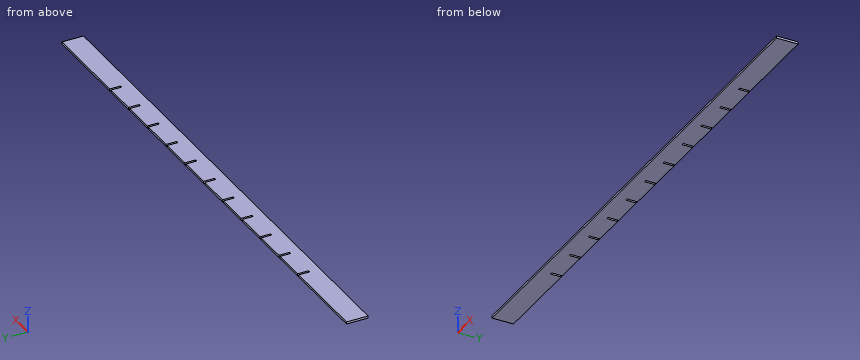
from build123d import *

# Parameters (mm, degrees)
ESQUISSE1_W                = 500
ESQUISSE1_H                = 20
BOSS_EXTRU_1_DEPTH         = 1
ESQUISSE2_W                = 2
ESQUISSE2_H                = 10
ENL_V_MAT_EXTRU_1_DEPTH    = 3
R_P_TITION_LIN_AIRE3_COUNT = 6
R_P_TITION_LIN_AIRE3_PITCH = 33
SYM_TRIE1_COPY_1_SKETCH_W  = 2
SYM_TRIE1_COPY_1_SKETCH_H  = 10
SYM_TRIE1_COPY_1_DEPTH     = 3
SYM_TRIE1_COPY_2_SKETCH_W  = 2
SYM_TRIE1_COPY_2_SKETCH_H  = 10
SYM_TRIE1_COPY_2_DEPTH     = 3
SYM_TRIE1_COPY_3_SKETCH_W  = 2
SYM_TRIE1_COPY_3_SKETCH_H  = 10
SYM_TRIE1_COPY_3_DEPTH     = 3
SYM_TRIE1_COPY_4_SKETCH_W  = 2
SYM_TRIE1_COPY_4_SKETCH_H  = 10
SYM_TRIE1_COPY_4_DEPTH     = 3
SYM_TRIE1_COPY_5_SKETCH_W  = 2
SYM_TRIE1_COPY_5_SKETCH_H  = 10
SYM_TRIE1_COPY_5_DEPTH     = 3
SYM_TRIE1_COPY_6_SKETCH_W  = 2
SYM_TRIE1_COPY_6_SKETCH_H  = 10
SYM_TRIE1_COPY_6_DEPTH     = 3


with BuildPart() as part:
    # Esquisse1 → Boss.-Extru.1 (new body, symmetric)
    with BuildSketch(Plane.XY):
        Rectangle(ESQUISSE1_W, ESQUISSE1_H)
    extrude(amount=BOSS_EXTRU_1_DEPTH, both=True)

    # Esquisse2 → Enlèv. mat.-Extru.1 (cut, through all)
    with BuildSketch(Plane.XY.offset(1)):
        with Locations((0, 5)):
            Rectangle(ESQUISSE2_W, ESQUISSE2_H)
    enl_v_mat_extru_1 = extrude(amount=-ENL_V_MAT_EXTRU_1_DEPTH, mode=Mode.SUBTRACT)

    # Répétition linéaire3: Enlèv. mat.-Extru.1 ×6
    with Locations(*[(-i * R_P_TITION_LIN_AIRE3_PITCH, 0, 0) for i in range(1, R_P_TITION_LIN_AIRE3_COUNT)]):
        add(enl_v_mat_extru_1, mode=Mode.SUBTRACT)

    # Symétrie1 copy 1 sketch → Symétrie1 copy 1 (cut, through all)
    with BuildSketch(Plane(origin=(33, 0, 1), x_dir=(-1, 0, 0), z_dir=(0, 0, 1))):
        with Locations((0, -5)):
            Rectangle(SYM_TRIE1_COPY_1_SKETCH_W, SYM_TRIE1_COPY_1_SKETCH_H)
    extrude(amount=-SYM_TRIE1_COPY_1_DEPTH, mode=Mode.SUBTRACT)

    # Symétrie1 copy 2 sketch → Symétrie1 copy 2 (cut, through all)
    with BuildSketch(Plane(origin=(66, 0, 1), x_dir=(-1, 0, 0), z_dir=(0, 0, 1))):
        with Locations((0, -5)):
            Rectangle(SYM_TRIE1_COPY_2_SKETCH_W, SYM_TRIE1_COPY_2_SKETCH_H)
    extrude(amount=-SYM_TRIE1_COPY_2_DEPTH, mode=Mode.SUBTRACT)

    # Symétrie1 copy 3 sketch → Symétrie1 copy 3 (cut, through all)
    with BuildSketch(Plane(origin=(99, 0, 1), x_dir=(-1, 0, 0), z_dir=(0, 0, 1))):
        with Locations((0, -5)):
            Rectangle(SYM_TRIE1_COPY_3_SKETCH_W, SYM_TRIE1_COPY_3_SKETCH_H)
    extrude(amount=-SYM_TRIE1_COPY_3_DEPTH, mode=Mode.SUBTRACT)

    # Symétrie1 copy 4 sketch → Symétrie1 copy 4 (cut, through all)
    with BuildSketch(Plane(origin=(132, 0, 1), x_dir=(-1, 0, 0), z_dir=(0, 0, 1))):
        with Locations((0, -5)):
            Rectangle(SYM_TRIE1_COPY_4_SKETCH_W, SYM_TRIE1_COPY_4_SKETCH_H)
    extrude(amount=-SYM_TRIE1_COPY_4_DEPTH, mode=Mode.SUBTRACT)

    # Symétrie1 copy 5 sketch → Symétrie1 copy 5 (cut, through all)
    with BuildSketch(Plane(origin=(165, 0, 1), x_dir=(-1, 0, 0), z_dir=(0, 0, 1))):
        with Locations((0, -5)):
            Rectangle(SYM_TRIE1_COPY_5_SKETCH_W, SYM_TRIE1_COPY_5_SKETCH_H)
    extrude(amount=-SYM_TRIE1_COPY_5_DEPTH, mode=Mode.SUBTRACT)

    # Symétrie1 copy 6 sketch → Symétrie1 copy 6 (cut, through all)
    with BuildSketch(Plane(origin=(0, 0, 1), x_dir=(-1, 0, 0), z_dir=(0, 0, 1))):
        with Locations((0, -5)):
            Rectangle(SYM_TRIE1_COPY_6_SKETCH_W, SYM_TRIE1_COPY_6_SKETCH_H)
    extrude(amount=-SYM_TRIE1_COPY_6_DEPTH, mode=Mode.SUBTRACT)


solid = part.part
Work out the finished part from the listing and answer in its coordinate system (mm). Give positions to 0.01 mm unless a question says otherwise; leave off trailing zeros. One line per item, written item: value. Start each with the question number.
1. Consider probe 1 along Y at (x, z) = (-66.5, 0.9). Determine where the line is inside the solid, lowest interval first.
2. Find section A-A (y = 6.25). State how many separate pieces and enclosed holes the cut face has, then the cut area to 3 significant figures.
3. Given pin 1 (8 mm diameter, centred on x = -98.5, y = 1, fed in from +Z), flat-ended and moving along its own axis, determine where the tip first touches the part or whether it passes through.
Geometry results:
1. probe 1: -10 to 0
2. separate pieces: 12
2. enclosed holes: 0
2. area: 956 mm2
3. pin 1: z = 1
